from build123d import *

# Parameters (mm, degrees)
F0_R     = 66.619234
F1_DEPTH = 15.24
F3_DEPTH = 17.78
F5_DEPTH = 25.4


with BuildPart() as f1:
    # F0 (on Top) → F1 (new body)
    with BuildSketch(Plane.XY):
        Circle(F0_R)
    extrude(amount=F1_DEPTH)

    # F2 (on face) → F3 (join)
    with BuildSketch(Plane.XY.offset(15.24)):
        Polygon((-39.33026, 39.587958), (-50.975195, 22.706943), (-55.735648, 2.759229), (-52.968692, -17.561134), (-43.048021, -35.509768), (-27.313476, -48.662612), (-7.890095, -55.2433), (12.598887, -54.363074), (31.386319, -46.140814), (45.934856, -31.686981), (54.279635, -12.953646), (55.293649, 7.52915), (48.83995, 26.995094), (35.790144, 42.8152), (17.906681, 52.852876), (-2.395178, 55.752479), (-22.373555, 51.1224), align=None)
    extrude(amount=F3_DEPTH)

    # F4 (on face) → F5 (join)
    with BuildSketch(Plane.XY.offset(33.02)):
        Polygon((-31.556715, -23.003328), (-17.251904, -35.033573), (1.005111, -39.038048), (19.031867, -34.099376), (32.698651, -21.348949), (38.874569, -3.707734), (36.144791, 14.782877), (25.134678, 29.88691), (8.366512, 38.144212), (-10.31832, 37.663134), (-26.63935, 28.553887), (-36.857626, 12.903288), (-38.632264, -5.703299), align=None)
    extrude(amount=F5_DEPTH)


solid = f1.part
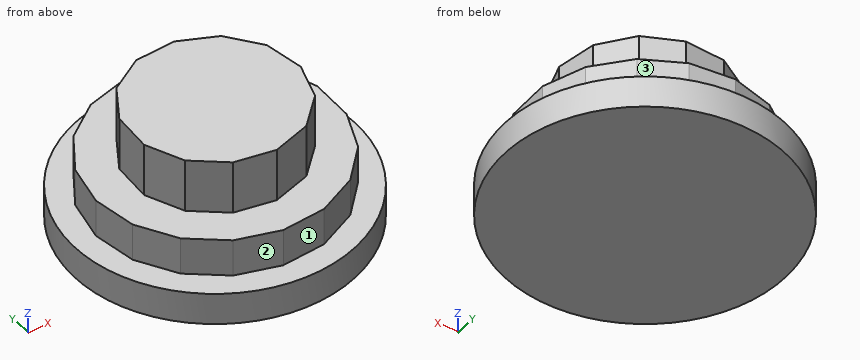
Could you check a few things on this model? Use its own coordinates, in mm. Face numbers are marked on the shaded views. A direction names the side the tool comes from. Round coordinates to 2 decimals unless told otherwise and drop trailing zeros. Order: outer loops, then holes, each group sorted by start corner. A loop starts at its lowest first (then second) coordinate and runs counter-clockwise, first axis right, second up.
(1) I'm going to push flat-ended pins straight in: pin 1 (3 mm diameter, centred on y = 3, z = 24, fed in from +X); pin 2 (6 mm diameter, centred on x = -34, y = -18, fed in from +Z); pin 3 (1.5 mm diameter, centred on x = -7, z = 31, fed in from +Y); pin 4 (10 mm diameter, centred on y = -23, z = 6, fed in from -X). Where does each tip first touch, or does it pass through?
Response values:
pin 1: stops at x = 55.14
pin 2: stops at z = 58.42
pin 3: stops at y = 54.86
pin 4: stops at x = -64.14
(2) Imagine slicing it at D-D (z = 24.5). Write out the boundary of the cut face in (x, y), plus the area to 3 significant figures.
Response values:
outline: (-55.74, 2.76) - (-52.97, -17.56) - (-43.05, -35.51) - (-27.31, -48.66) - (-7.89, -55.24) - (12.6, -54.36) - (31.39, -46.14) - (45.93, -31.69) - (54.28, -12.95) - (55.29, 7.53) - (48.84, 27) - (35.79, 42.82) - (17.91, 52.85) - (-2.4, 55.75) - (-22.37, 51.12) - (-39.33, 39.59) - (-50.98, 22.71) - close
area: 9,560 mm2
(3) Imagine slicing it at B-B (x = -25). Write out the boundary of the cut face in (y, z), plus the area to 3 significant figures.
Response values:
outline: (-61.75, 0) - (61.75, 0) - (61.75, 15.24) - (49.34, 15.24) - (49.34, 33.02) - (29.47, 33.02) - (29.47, 58.42) - (-28.52, 58.42) - (-28.52, 33.02) - (-49.45, 33.02) - (-49.45, 15.24) - (-61.75, 15.24) - close
area: 5,110 mm2
(4) Which directions (+Z, -Z, +X, -X, +Y, -Y) give clear straight access to the entire face, cutting with the end or side of a thin tool? Please do the marked faces 1, 2 and 3.
Response values:
face 1: +Z, +X, -Y
face 2: +Z, -X, -Y
face 3: +Z, +X, +Y
(5) Imagine slicing it at A-A (z = 39.5). Write out the boundary of the cut face in (x, y), plus the area to 3 significant figures.
Response values:
outline: (-38.63, -5.7) - (-31.56, -23) - (-17.25, -35.03) - (1.01, -39.04) - (19.03, -34.1) - (32.7, -21.35) - (38.87, -3.71) - (36.14, 14.78) - (25.13, 29.89) - (8.37, 38.14) - (-10.32, 37.66) - (-26.64, 28.55) - (-36.86, 12.9) - close
area: 4,610 mm2
(6) Please list where these lines run through material, in increasing order: line 1 along Z through (x, y) = (41.5, -51); line 2 along Z through (x, y) = (-30.5, 33); line 3 along X through (y, z) = (-7.5, 54).
Response values:
line 1: z = 0 to 15.24
line 2: z = 0 to 33.02
line 3: x = -37.9 to 37.55
(7) Imagine slicing it at C-C (y = 0). Write out the boundary of the cut face in (x, z), plus the area to 3 significant figures.
Response values:
outline: (-66.62, 0) - (66.62, 0) - (66.62, 15.24) - (54.92, 15.24) - (54.92, 33.02) - (38.33, 33.02) - (38.33, 58.42) - (-38.09, 58.42) - (-38.09, 33.02) - (-55.36, 33.02) - (-55.36, 15.24) - (-66.62, 15.24) - close
area: 5,930 mm2
